Autodesk Inventor part; units mm, degrees
ref_plane "YZ Plane" through (0, 0, 0) normal (1, 0, 0) x (0, 1, 0)
ref_plane "XZ Plane" through (0, 0, 0) normal (0, 1, 0) x (-1, 0, 0)
ref_plane "XY Plane" through (0, 0, 0) normal (0, 0, 1) x (1, 0, 0)
sketch "스케치1" plane through (0, 0, 0) normal (0, 1, 0) x (-1, 0, 0)
  line L0 (0, 0) -> (0, -14)
  line L1 (0, -14) -> (10.4, -14)
  line L2 (0, 0) -> (10.4, 0)
  line L3 (10.4, 0) -> (10.4, -1.8)
  line L4 (10.4, -1.8) -> (5.2, -1.8)
  line L5 (5.2, -1.8) -> (5.2, -5.5)
  line L6 (5.2, -5.5) -> (4.4, -5.5)
  line L7 (4.4, -5.5) -> (4.4, -8.5)
  line L8 (4.4, -8.5) -> (5.2, -8.5)
  line L9 (5.2, -8.5) -> (5.2, -12.2)
  line L10 (5.2, -12.2) -> (10.4, -12.2)
  line L11 (10.4, -12.2) -> (10.4, -14)
  line L12 (10.4, -0.95) -> (4.4, -0.95) construction
  line L13 (4.4, -0.95) -> (4.4, -13.05) construction
  line L14 (4.4, -13.05) -> (10.4, -13.05) construction
  dimension "d0" = 14
  dimension "d2" = 10.4
  dimension "d3" = 1.8
  dimension "d5" = 3.7
  dimension "d6" = 0.8
  dimension "d7" = 3
  dimension "d8" = 0.8
  dimension "d9" = 3.7
  dimension "d47" = 12.1
  dimension "d48" = 0.85
  dimension "d49" = 0.85
  dimension "d63" = 6
extrude "돌출1" add sketch "스케치1" along normal blind 4
sketch "스케치9" plane through (-10.4, 0, -14) normal (-1, 0, 0) x (0, 0, 1)
  line L0 (12.2, 0) -> (14, 0)
  line L1 (14, 0) -> (14, 4)
  line L2 (12.2, 4) -> (14, 4)
  line L3 (12.2, 0) -> (12.2, 4)
  line L4 (0, 0) -> (1.8, 0)
  line L5 (1.8, 0) -> (1.8, 4)
  line L6 (0, 4) -> (1.8, 4)
  line L7 (0, 0) -> (0, 4)
  line L8 (13.05, 1.5) -> (0.95, 1.5)
  line L9 (0.95, 1.5) -> (0.95, 2.5)
  line L10 (0.95, 2.5) -> (13.05, 2.5)
  line L11 (13.05, 2.5) -> (13.05, 1.5)
  dimension "d55" = 0.95
  dimension "d56" = 0.95
  dimension "d60" = 1
  dimension "d61" = 1.5
  dimension "d62" = 1.5
  dimension "d71" = 12.1
extrude "돌출9" cut sketch "스케치9" against normal blind 6 contours L8 L5 L10 L3 | L3 L10 L11 L8 | L8 L9 L10 L5
sketch "스케치10" plane through (0, 4, 0) normal (0, 1, 0) x (1, 0, 0)
  line L0 (0, 0) -> (0, 14)
  line L1 (0, 14) -> (-10.4, 14)
  line L2 (-10.4, 14) -> (-10.4, 12.2)
  line L3 (-10.4, 12.2) -> (-5.2, 12.2)
  line L4 (-5.2, 12.2) -> (-5.2, 8.5)
  line L5 (-5.2, 8.5) -> (-4.4, 8.5)
  line L6 (-4.4, 8.5) -> (-4.4, 5.5)
  line L7 (-4.4, 5.5) -> (-5.2, 5.5)
  line L8 (-5.2, 5.5) -> (-5.2, 1.8)
  line L9 (-5.2, 1.8) -> (-10.4, 1.8)
  line L10 (-10.4, 1.8) -> (-10.4, 0)
  line L11 (-10.4, 0) -> (0, 0)
  line L12 (-5.2, 1.8) -> (-10.4, 1.8)
  line L13 (-5.2, 12.2) -> (-10.4, 12.2)
  line L14 (-10.4, 1.8) -> (-9.4, 1.8)
  line L15 (-9.4, 1.8) -> (-9.4, 12.2)
  line L16 (-9.4, 12.2) -> (-10.4, 12.2)
  line L17 (-10.4, 12.2) -> (-10.4, 1.8)
  point P0 (-9.4, 1.8)
  point P1 (-9.4, 12.2)
  dimension "d64" = 1
extrude "돌출10" add sketch "스케치10" against normal up to surface (1.5 mm away) contours L17 L3 L15 L9
sketch "스케치11" plane through (0, 4, 0) normal (0, 1, 0) x (1, 0, 0)
  line L0 (-9.4, 1.3) -> (-5.2, 1.3)
  line L1 (-5.2, 1.3) -> (-5.2, 12.7)
  line L2 (-5.2, 12.7) -> (-9.4, 12.7)
  line L3 (-9.4, 12.7) -> (-9.4, 1.3)
  line L4 (-9.4, 1.8) -> (-9.4, 12.2)
  line L5 (-5.2, 12.2) -> (-5.2, 8.5)
  line L6 (-5.2, 1.8) -> (-9.4, 1.8)
  line L7 (-9.4, 12.2) -> (-5.2, 12.2)
  point P0 (0, 0)
  point P1 (-5.2, 12.2)
  dimension "d67" = 0.5
  dimension "d68" = 0.5
extrude "돌출11" cut sketch "스케치11" against normal up to surface (1.5 mm away) contours L3 L6 L1 L0 | L3 L2 L1 L7
equation "\"d5\" = d9"
equation "\"d9\" = 0.5 * d0 - 0.5 * d7 - d3"
equation "\"d48\" = d49"
equation "\"d55\" = d56"
equation "\"d61\" = d62"
properties part number "_3D 인쇄"
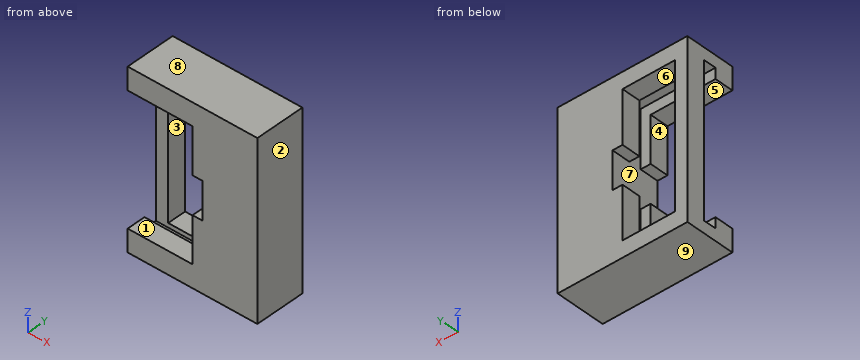
Source: CAD feature listing. Evaluate the final solid. Frame: model axes, mm. Face numbers are marked on the shaded views. A direction names the side the tool comes from. Coordinates: 2 decimals unless noted, no trailing zeros. Loops run counter-clockwise (first coordinate to the right, second up) from the corner with the lowest first, then second, coordinate; pieces in that order, holes last. Notation, with made-up numbers: (-38, -12.5) -> (-30, -12.5) arc R20 ccw to (-30, 0.5) -> close; hole circle Ø9 at (-12.5, 14.25). An arc over 180 degrees is marked (long way). One line per item, written item: value. Start each with the question number.
Q1. Set-up query: the marked faces 5, 6, 7, 8 and 9. Return all of +Z, -Z, +X, -X, +Y, -Y with unobstructed straight access to the full face (end or side cutting, diameter ignored); none if empty.
Q2. Section query D-D, the plane y = 0.85. Return the cut outline in (x, z).
Q3. Line query: line 1 along Z through (x, y) = (-4.5, 0.45); line 2 along Z through (x, y) = (-7.75, 0.3); line 3 along X through (y, z) = (2.95, -3). Output: solid intervals per line, ascending.
Q4. Contact query for a flat-ended pin moving along its axis: P1, Ø1.6, axis at y = 0.5, z = -3.5, coming from the -X side. Output: stop coordinate, or through.
Q5. Section query A-A, the plane z = -8.25. Return the cut outline in (x, y), and give its area (3 significant figures).
Q6. Mould query, pull axis X, two halves, no side actions, for the marked faces 1, 2, 3 and 4. Classes: pulls with the +X half, pulls with the -X half, needs draft (parallel to the pull), parting line crosses it, or undercut.
Q7. Section query C-C, the plane x = -9.25. Return the cut outline in (y, z), and give its area (3 significant figures).
Q8. Section query B-B, the plane y = 3.5. Return the cut outline in (x, z).
Results:
1. face 5: -X, -Y
1. face 6: +Y
1. face 7: none
1. face 8: +Z, +X, -X, +Y, -Y
1. face 9: -Z, +X, -X, +Y, -Y
2. outline: (-10.4, -14) -> (0, -14) -> (0, 0) -> (-10.4, 0) -> (-10.4, -1.8) -> (-5.2, -1.8) -> (-5.2, -5.5) -> (-4.4, -5.5) -> (-4.4, -8.5) -> (-5.2, -8.5) -> (-5.2, -12.2) -> (-10.4, -12.2) -> close
3. line 1: -14 to -8.5, -5.5 to 0
3. line 2: -14 to -12.2, -1.8 to 0
3. line 3: -10.4 to -9.4, -5.2 to 0
4. P1: x = -5.2
5. outline: (-10.4, 2.5) -> (-9.4, 2.5) -> (-9.4, 4) -> (-10.4, 4) -> close; (-4.4, 0) -> (0, 0) -> (0, 4) -> (-4.4, 4) -> close
5. area: 19.1 mm^2
6. face 1: needs draft
6. face 2: pulls with the +X half
6. face 3: undercut
6. face 4: pulls with the -X half
7. outline: (0, -14) -> (4, -14) -> (4, -12.7) -> (2.5, -12.7) -> (2.5, -13.05) -> (1.5, -13.05) -> (1.5, -12.2) -> (0, -12.2) -> close; (0, -1.8) -> (1.5, -1.8) -> (1.5, -0.95) -> (2.5, -0.95) -> (2.5, -1.3) -> (4, -1.3) -> (4, 0) -> (0, 0) -> close
7. area: 11.2 mm^2
8. outline: (-10.4, -14) -> (0, -14) -> (0, 0) -> (-10.4, 0) -> close; hole (-9.4, -12.7) -> (-5.2, -12.7) -> (-5.2, -8.5) -> (-4.4, -8.5) -> (-4.4, -5.5) -> (-5.2, -5.5) -> (-5.2, -1.3) -> (-9.4, -1.3) -> close
